Geometry: see drawing. Coordinates: mm, zero at the bounding-box minimum. A direction names the side the tool comes from. Give positions to 0.01 mm unless a question says otherwise; leave off trailing zeros. Order: outer loops, then holes, each group sorted by start corner. A loop starts at its lowest first (then second) coordinate and runs counter-clockwise, first axis right, second up. Notation, with made-up numbers: M -19.5,34 L 25.5,34 A31 ccw 25.5,68 Z; hole C -5,44 d2. An arc over 180 degrees is marked long. Return JSON: item names as keys, results as strings.
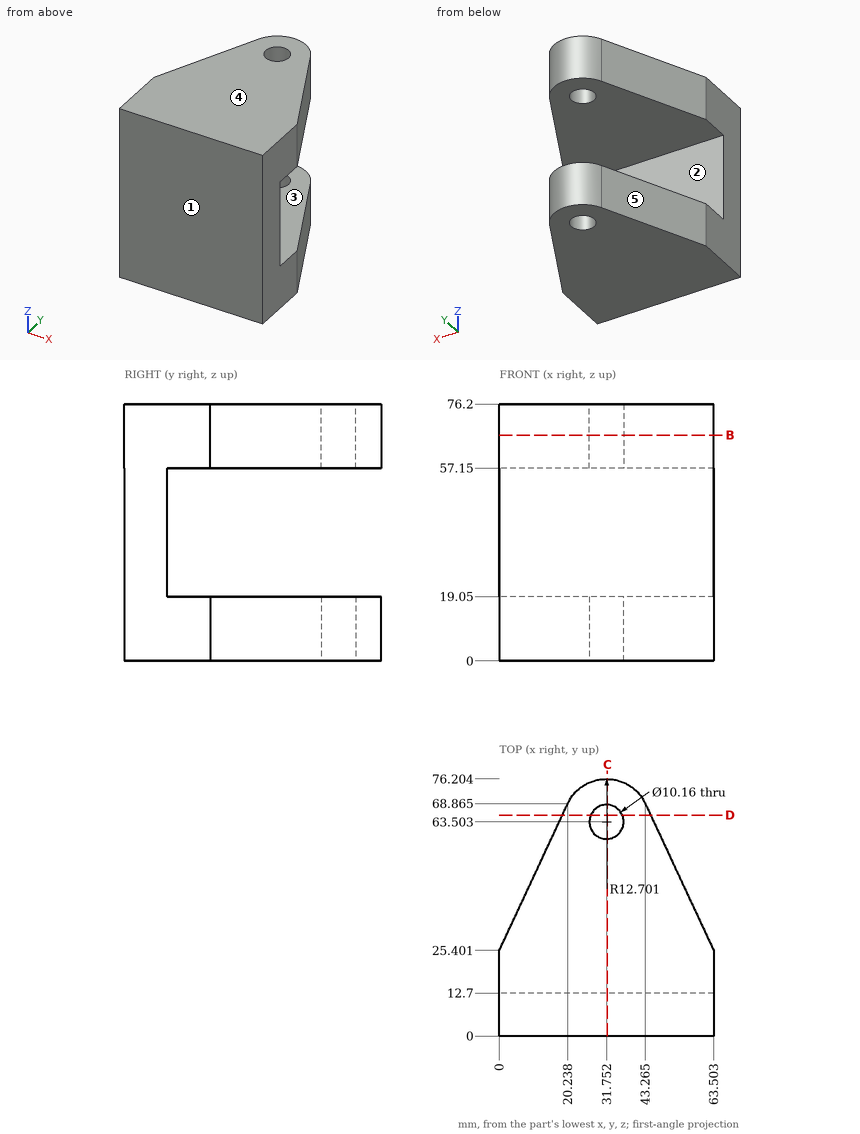
1. Ray query, probe 1 along Z at (x, y) = (59.5, 18); probe 2 along Y at (x, z) = (31.5, 69.5); probe 3 along Y at (x, z) = (37.5, 43.5). Return the intervals inside material, ascending.
Evaluation:
{"probe 1": "z = 0 to 19.05, 57.15 to 76.2", "probe 2": "y = 0 to 58.43, 68.58 to 76.2", "probe 3": "y = 0 to 12.7"}
2. Section query B-B (z = 67). Return loops of the section in (x, y) (1 decimal).
Evaluation:
{"outline": "M 0,0 L 63.5,0 L 63.5,25.4 L 43.3,68.9 A12.7 ccw 20.2,68.9 L 0,25.4 Z; hole C 31.8,63.5 d10.2"}
3. Set-up query: the marked faces 1 and 2. Return all of +Z, -Z, +X, -X, +Y, -Y with unobstructed straight access to the full face (end or side cutting, diameter ignored); none if empty.
Evaluation:
{"face 1": "+Z, -Z, +X, -X, -Y", "face 2": "+X, -X, +Y"}
4. Section query C-C (x = 32). Return loops of the section in (y, z), then the cut area to 3 significant figures.
Evaluation:
{"outline": "M 0,0 L 58.43,0 L 58.43,19.05 L 12.7,19.05 L 12.7,57.15 L 58.43,57.15 L 58.43,76.2 L 0,76.2 Z; M 68.58,0 L 76.2,0 L 76.2,19.05 L 68.58,19.05 Z; M 68.58,57.15 L 76.2,57.15 L 76.2,76.2 L 68.58,76.2 Z", "area": "3,000 mm^2"}
5. Draft query along Z for the marked faces 3, 4 and 5. Return one class per face: pulls with the +Z half, pulls with the -Z half, needs draft (parallel to the pull), parting line crosses it, or undercut.
Evaluation:
{"face 3": "undercut", "face 4": "pulls with the +Z half", "face 5": "needs draft"}
6. First-contact query: pin 1 (10 mm diameter, centred on y = 44, z = 17.5, fed in from -X); pin 2 (4 mm diameter, centred on x = 18, z = 60, fed in from +Y) (1 decimal). Flat tips, straight axial feed; report the tip coordinate or a pass-through.
Evaluation:
{"pin 1": "stops at x = 6.33", "pin 2": "stops at y = 68.4"}
7. Section query D-D (y = 65.5). Return loops of the section in (x, z), then the cut area to 3 significant figures.
Evaluation:
{"outline": "M 18.67,0 L 27.08,0 L 27.08,19.05 L 18.67,19.05 Z; M 18.67,57.15 L 27.08,57.15 L 27.08,76.2 L 18.67,76.2 Z; M 36.42,0 L 44.83,0 L 44.83,19.05 L 36.42,19.05 Z; M 36.42,57.15 L 44.83,57.15 L 44.83,76.2 L 36.42,76.2 Z", "area": "641 mm^2"}
